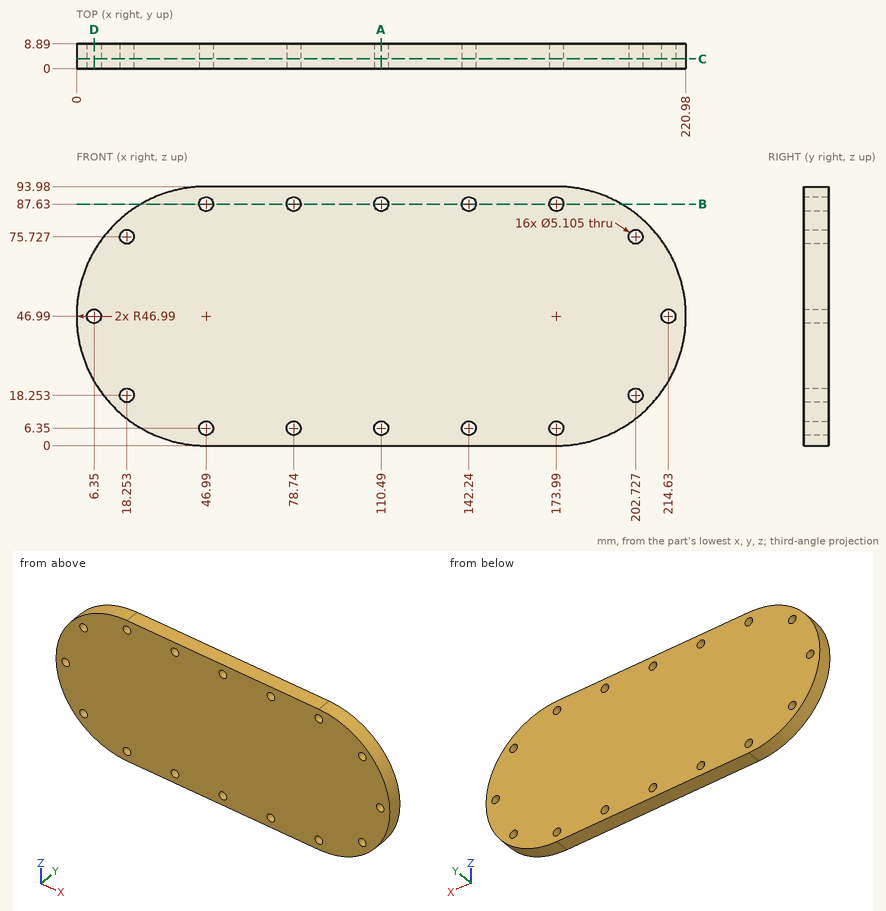
Could you check a few things on this drawing? It's one solid part, dimensions in mm from its lowest x, y, z. Coordinates: 2 decimals unless noted, no trailing zeros. Order: outer loops, then holes, each group sorted by start corner. A loop starts at its lowest first (then second) coordinate and runs counter-clockwise, first axis right, second up. Notation, with made-up numbers: M 54.25,-40 L 83.25,-40 A14 ccw 83.25,-36 Z; hole C 67.5,13.25 d1. An arc over 180 degrees is marked long. Use one line per item in the form item = value. Start each with the question number.
1. Please list where these lines run through material, in increasing order: line 1 (X direction, y = 3.25, z = 46.99); line 2 (Z direction, x = 173.99, y = 5.75); line 3 (X direction, y = 4.5, z = 45.5) (1 decimal).
2. Suppose I cut it at B-B on z = 87.63. Write out the boundary of the cut face in (x, y), then the cut area to 3 significant figures.
3. Suppose I cut it at C-C on y = 3.5. Count the separate pieces of the cut face and the enclosed holes in it, then the cut area to 3 significant figures.
4. Suppose I cut it at A-A on x = 110.49. Write out the boundary of the cut face in (y, z).
5. For pin 1 (4 mm diameter, centred on y = 5.5, z = 58.5, fed in from -X); pin 2 (2 mm diameter, centred on x = 127.5, z = 81, fed in from -Y); pin 3 (4 mm diameter, centred on y = 6.5, z = 39.5, fed in from -X); pin 4 (2 mm diameter, centred on y = 7.5, z = 68, fed in from -X), each with a flat end and sliding along its axis, tell me the tip position at first contact or that it passes through.
6. Suppose I cut it at D-D on x = 6.35. Write out the boundary of the cut face in (y, z), then the cut area to 3 significant figures.
Geometry says:
q1.line_1 = 0 to 3.8, 8.9 to 212.08, 217.18 to 220.98
q1.line_2 = 0 to 3.8, 8.9 to 85.08, 90.18 to 93.98
q1.line_3 = 0 to 4.3, 8.4 to 212.6, 216.7 to 221
q2.outline = M 23.4,0 L 44.44,0 L 44.44,8.89 L 23.4,8.89 Z; M 49.54,0 L 76.19,0 L 76.19,8.89 L 49.54,8.89 Z; M 81.29,0 L 107.94,0 L 107.94,8.89 L 81.29,8.89 Z; M 113.04,0 L 139.69,0 L 139.69,8.89 L 113.04,8.89 Z; M 144.79,0 L 171.44,0 L 171.44,8.89 L 144.79,8.89 Z; M 176.54,0 L 197.58,0 L 197.58,8.89 L 176.54,8.89 Z
q2.area = 1,320 mm^2
q3.separate_pieces = 1
q3.enclosed_holes = 16
q3.area = 18,500 mm^2
q4.outline = M 0,0 L 8.89,0 L 8.89,3.8 L 0,3.8 Z; M 0,8.9 L 8.89,8.9 L 8.89,85.08 L 0,85.08 Z; M 0,90.18 L 8.89,90.18 L 8.89,93.98 L 0,93.98 Z
q5.pin_1 = 0.97
q5.pin_2 = 0
q5.pin_3 = 0.32
q5.pin_4 = 4.47
q6.outline = M 0,23.4 L 8.89,23.4 L 8.89,44.44 L 0,44.44 Z; M 0,49.54 L 8.89,49.54 L 8.89,70.58 L 0,70.58 Z
q6.area = 374 mm^2
